Verification items for this drawing (mm, ordinates from the low corner). Round coordinates to 2 decimals unless told otherwise and drop trailing zeros. Answer in a Markdown table with one row per item. Add a question column.
1. Sectioned sample at A-A, the plane y = 21.75. Count the separate pieces of the cut face and the enclosed holes in it, then the cut area to 3 significant figures.
2. Draft check along X on the marked faces 1, 2, 3 and 4. Enter one of: +X half, -X half, draft (parallel to the pull), parting line (faces both ways), or undercut.
3. Depth check by flat-ended pin: P1, Ø2.5, axis at x = 57.5, z = 6, coming from the +Y side. Enter the tip coordinate at first touch or a pass-through.
4. Material ranges on L1, parallel to Y at x = 19.5, z = 4 (1 decimal); L2, parallel to Z at x = 119, y = 20.25 (1 decimal); L3, parallel to Z at x = 117.5, y = 21 (1 decimal), recorded low to high. Write a range as from..to.
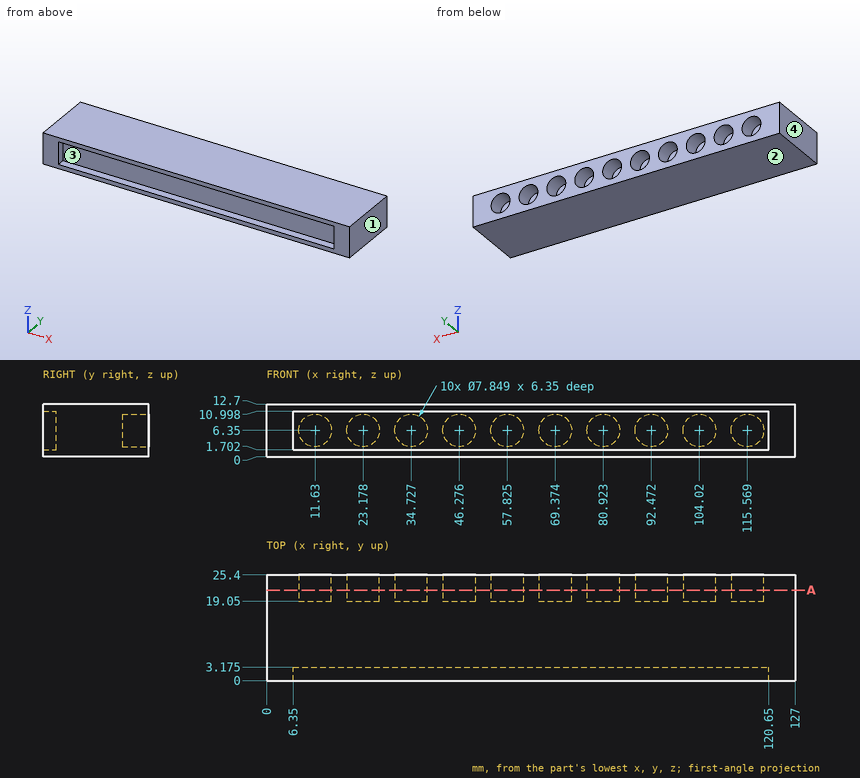
Answer key:
| question | item | result |
|---|---|---|
| 1 | separate pieces | 1 |
| 1 | enclosed holes | 10 |
| 1 | area | 1,130 mm² |
| 2 | face 1 | +X half |
| 2 | face 2 | draft |
| 2 | face 3 | undercut |
| 2 | face 4 | -X half |
| 3 | P1 | stops at y = 19.05 |
| 4 | L1 | y = 3.2..25.4 |
| 4 | L2 | z = 0..4.4, 8.3..12.7 |
| 4 | L3 | z = 0..2.9, 9.8..12.7 |
